Geometry: final body of the model. Coordinates: model frame, mm. Face numbers are marked on the shaded views. A direction names the side the tool comes from. Coordinates: 2 decimals unless noted, no trailing zeros. Order: outer loops, then holes, each group sorted by start corner. A loop starts at its lowest first (then second) coordinate and runs counter-clockwise, first axis right, second up. Notation, with made-up numbers: M -15,-33 L 9,-33 A17 ccw 9,-12 Z; hole C -9,45 d6. An arc over 180 degrees is marked long. One line per question, with ' | ' between items.
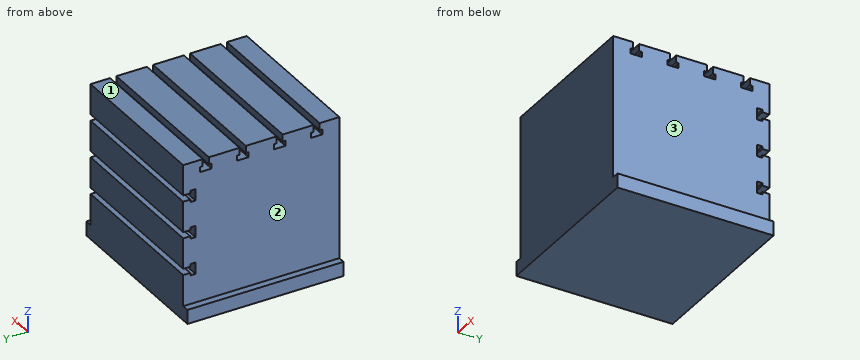
from build123d import *

# Parameters (mm, degrees)
BOSS_EXTRUDE1_DEPTH = 550
CUT_EXTRUDE1_REACH  = 969.277
CUT_EXTRUDE2_REACH  = 969.277
LPATTERN1_COUNT     = 3
LPATTERN1_PITCH     = 130
LPATTERN2_COUNT     = 4
LPATTERN2_PITCH     = 130


with BuildPart() as part:
    # Sketch1 → Boss-Extrude1 (new body)
    with BuildSketch(Plane(origin=(0, 0, 0), x_dir=(1, 0, 0), z_dir=(0, 1, 0))):
        Polygon((300, 0), (-300, 0), (-300, -50), (-275, -50), (-275, -550), (275, -550), (275, -50), (300, -50), align=None)
    extrude(amount=-BOSS_EXTRUDE1_DEPTH)

    # Sketch2 → Cut-Extrude1 (cut, up to next)
    with BuildSketch(Plane.ZY.offset(275), mode=Mode.PRIVATE) as cut_extrude1_sk1:
        Polygon((442.4, 0), (442.4, -24.8), (451.6, -24.8), (451.6, -43), (411.2, -43), (411.2, -24.8), (420.4, -24.8), (420.4, 0), align=None)
    cut_extrude1_tool1 = extrude(cut_extrude1_sk1.sketch, amount=-CUT_EXTRUDE1_REACH, mode=Mode.PRIVATE) & part.part
    cut_extrude1 = cut_extrude1_tool1.solids().sort_by_distance((-275, -24.741921, 431.4))[0]
    add(cut_extrude1, mode=Mode.SUBTRACT)

    # Sketch3 → Cut-Extrude2 (cut, up to next)
    with BuildSketch(Plane.ZY.offset(275), mode=Mode.PRIVATE) as cut_extrude2_sk1:
        Polygon((550, -90.5), (550, -68.5), (525.2, -68.5), (525.2, -59.3), (507, -59.3), (507, -99.7), (525.2, -99.7), (525.2, -90.5), align=None)
    cut_extrude2_tool1 = extrude(cut_extrude2_sk1.sketch, amount=-CUT_EXTRUDE2_REACH, mode=Mode.PRIVATE) & part.part
    cut_extrude2 = cut_extrude2_tool1.solids().sort_by_distance((-275, -79.5, 525.258079))[0]
    add(cut_extrude2, mode=Mode.SUBTRACT)

    # LPattern1: Cut-Extrude1 ×3
    with Locations(*[(0, 0, -i * LPATTERN1_PITCH) for i in range(1, LPATTERN1_COUNT)]):
        add(cut_extrude1, mode=Mode.SUBTRACT)

    # LPattern2: Cut-Extrude2 ×4
    with Locations(*[(0, -i * LPATTERN2_PITCH, 0) for i in range(1, LPATTERN2_COUNT)]):
        add(cut_extrude2, mode=Mode.SUBTRACT)


solid = part.part
1. Pin query (flat end, axial travel): P1, Ø7.5, axis at x = -102.5, y = -483.5, coming from the -Z side; P2, Ø7.5, axis at x = -284.5, y = -361, coming from the +Z side; P3, Ø2, axis at y = -325.5, z = 329.5, coming from the -X side. Return the tip coordinate at first contact, or that it passes through.
Response values:
P1: stops at z = 0 | P2: stops at z = 50 | P3: stops at x = -275
2. Section A-A, the plane y = -513. Output: boundary loops of the cut face in (x, z), and give its area (3 significant figures).
Response values:
outline: M -300,0 L 300,0 L 300,50 L 275,50 L 275,550 L -275,550 L -275,50 L -300,50 Z | area: 305,000 mm^2
3. Section B-B, the plane z = 89. Output: boundary loops of the cut face in (x, y), and give its area (4 significant figures).
Response values:
outline: M -275,-550 L 275,-550 L 275,0 L -275,0 Z | area: 302,500 mm^2
4. Section D-D, the plane z = 169. Output: boundary loops of the cut face in (x, y), and give its area (3 significant figures).
Response values:
outline: M -275,-550 L 275,-550 L 275,-43 L -275,-43 Z | area: 279,000 mm^2
5. Material intervals for line 1 (Z direction, x = -261, y = -32); line 2 (Z direction, x = 11, y = -99); line 3 (Y direction, x = 63, z = 284.5), sorted ascending. Write a range as [from, to].
Response values:
line 1: z = [0, 151.2], [191.6, 281.2], [321.6, 411.2], [451.6, 550] | line 2: z = [0, 507], [525.2, 550] | line 3: y = [-550, -43], [-24.8, 0]
6. Access query for the marked faces 1, 2 and 3. Directions: +Z, -Z, +X, -X, +Y, -Y. A direction counts if a zero-diameter tool reaches every point of the face in a straight line with its end or side. Return the directions, or none.
Response values:
face 1: +Z, +X, -X, +Y, -Y | face 2: +Z, -X, +Y, -Y | face 3: +Z, +X, +Y, -Y
7. Section C-C, the plane y = -206.5. Output: boundary loops of the cut face in (x, z), and give its area (3 significant figures).
Response values:
outline: M -300,0 L 300,0 L 300,50 L 275,50 L 275,507 L -275,507 L -275,50 L -300,50 Z | area: 281,000 mm^2
